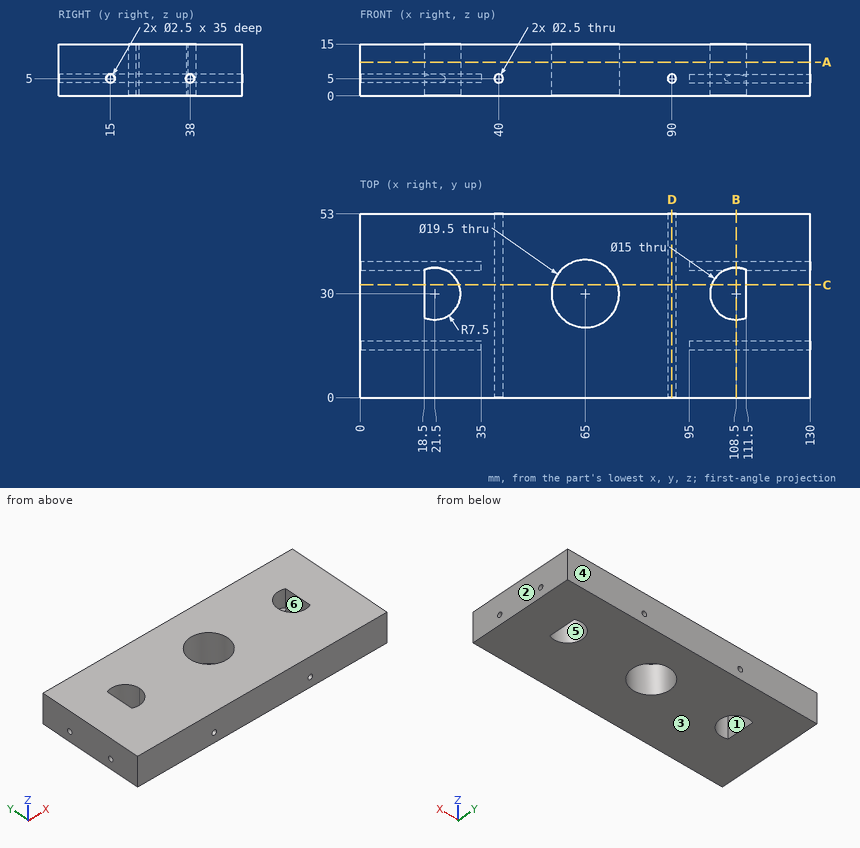
Source: three-view drawing plus pictorial views. Frame: mm from the lowest corner of the part. A direction names the side the tool comes from. Give positions to 0.01 mm unless a question says otherwise; leave off trailing zeros. Order: outer loops, then holes, each group sorted by start corner. A loop starts at its lowest first (then second) coordinate and runs counter-clockwise, first axis right, second up.
1. Section D-D on x = 90. Return the cut outline in (y, z), and give its area (4 significant figures).
Derived:
outline: (0, 0) - (53, 0) - (53, 3.75) - (0, 3.75) - close; (0, 6.25) - (53, 6.25) - (53, 15) - (0, 15) - close
area: 662.5 mm2
2. Material intervals for L1, parallel to Z at x = 112, y = 38; L2, parallel to X at y = 32.5, z = 13; L3, parallel to Y at x = 108.5, z = 11.75, sorted ascending.
Derived:
L1: z = 0 to 3.75, 6.25 to 15
L2: x = 0 to 18.5, 28.57 to 55.58, 74.42 to 101.43, 111.5 to 130
L3: y = 0 to 22.5, 37.5 to 53
3. Pin query (flat end, axial travel): pin 1 (1.5 mm diameter, centred on y = 15, z = 5, fed in from +X); pin 2 (0.8 mm diameter, centred on y = 38.5, z = 5.5, fed in from -X). Return the tip coordinate at first contact, or that it passes through.
Derived:
pin 1: stops at x = 95
pin 2: stops at x = 35
4. Section A-A on z = 9.75. Return the cut outline in (x, y).
Derived:
outline: (0, 0) - (130, 0) - (130, 53) - (0, 53) - close; hole (18.5, 23.13) arc R7.5 ccw to (29, 30) arc R7.5 ccw to (18.5, 36.87) - close; hole circle Ø19.5 at (65, 30); hole (111.5, 23.13) - (111.5, 36.87) arc R7.5 ccw (long way) to start
5. Reachability of the marked faces 1 and 2 from +Z, -Z, +X, -X, +Y, -Y: full face, straight path, thin tool, end or side. Return the list, or none.
Derived:
face 1: +Z, -Z
face 2: +Z, -Z, +X, +Y, -Y
6. Section B-B on x = 108.5. Return the cut outline in (y, z).
Derived:
outline: (0, 0) - (22.5, 0) - (22.5, 15) - (0, 15) - close; (37.5, 0) - (53, 0) - (53, 15) - (37.5, 15) - (37.5, 6.15) arc R1.25 cw (long way) to (37.5, 3.85) - close; hole circle Ø2.5 at (15, 5)
7. Section C-C on y = 32.5. Return the cut outline in (x, z).
Derived:
outline: (0, 0) - (18.5, 0) - (18.5, 15) - (0, 15) - close; (28.57, 0) - (55.58, 0) - (55.58, 15) - (28.57, 15) - close; (74.42, 0) - (101.43, 0) - (101.43, 15) - (74.42, 15) - close; (111.5, 0) - (130, 0) - (130, 15) - (111.5, 15) - close; hole circle Ø2.5 at (40, 5); hole circle Ø2.5 at (90, 5)
8. Mould query, pull axis Y, two halves, no side actions, for the marked faces 3, 4, 5 and 6. Classes: released by +Y, released by -Y, zero draft, split by the parting line, or undercut.
Derived:
face 3: zero draft
face 4: released by +Y
face 5: undercut
face 6: undercut
